For this review, take the finished solid that the model builds, in its own axes (mm). Coordinates: 2 decimals unless noted, no trailing zeros. Loops run counter-clockwise (first coordinate to the right, second up) from the corner with the lowest first, then second, coordinate; pieces in that order, holes last. Notation, with made-up numbers: M -29,61 L -5,61 A34 cw -5,100 Z; hole C 15,66.5 d8. An arc over 180 degrees is marked long. Put each result on its own line as item: value.
```python
from build123d import *

# Parameters (mm, degrees)
F1_DEPTH      = 3.414395
F1_DEPTH_BACK = 3.414395
F3_D          = 5.08
F3_DEPTH      = 38.1
F3_TIP        = 1.5261859723
F4_R          = 2.54


with BuildPart() as f1:
    # F0 (on Top) → F1 (new body, two sides)
    with BuildSketch(Plane.XY) as f1_sk:
        Polygon((27.5532683375, 33.9854207361), (8.2568451762, 33.9854207361), (8.2568451762, 27.1566307361), (62.6822561026, 27.1566307361), (81.9869935513, 27.1566307361), (81.9869935513, 33.9854207361), (78.0837014318, 33.9854207361), (71.3711140723, 33.9854207361), (58.8463247403, 33.9854207361), (56.5806804269, 33.9854207361), (53.2887220937, 33.9854207361), (51.0230777803, 33.9854207361), (45.4654522794, 33.9854207361), (43.199807966, 33.9854207361), (37.6421824652, 33.9854207361), (35.3765381518, 33.9854207361), (29.8189126509, 33.9854207361), align=None)
    extrude(amount=F1_DEPTH)
    extrude(f1_sk.sketch, amount=-F1_DEPTH_BACK)

    # F3
    with Locations(Plane.YZ.offset(81.9869935513)):
        with Locations((30.5710257361, 0)):
            Hole(F3_D / 2, depth=F3_DEPTH)
            with Locations((0, 0, -(F3_DEPTH + F3_TIP / 2))):  # 118° drill point
                Cone(0, F3_D / 2, F3_TIP, mode=Mode.SUBTRACT)

    # F4
    f4_edges = [f1.edges().sort_by_distance(p)[0] for p in [
        (45.121919, 33.985421, 3.414395),
        (45.121919, 27.156631, 3.414395),
        (45.121919, 33.985421, -3.414395),
        (45.121919, 27.156631, -3.414395),
    ]]
    fillet(f4_edges, radius=F4_R)


solid = f1.part
```
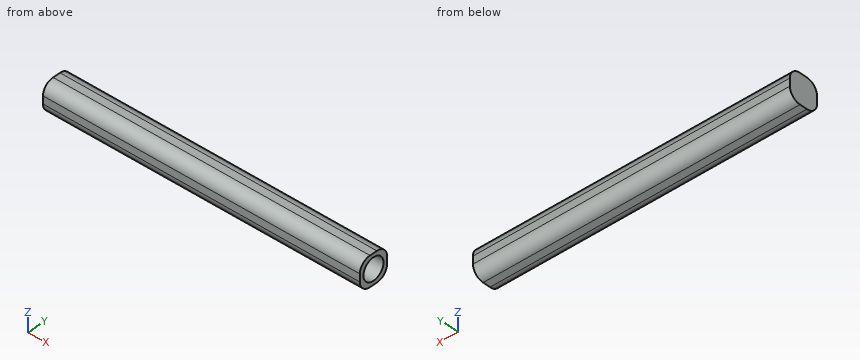
(1) Add section B-B (x = 39). Write out the cut boundary in (y, z), plus the area to 3 significant figures.
Determined:
outline: M 27.16,-0.87 A2.54 ccw 29.7,-3.41 L 31.45,-3.41 A2.54 ccw 33.99,-0.87 L 33.99,0.87 A2.54 ccw 31.45,3.41 L 29.7,3.41 A2.54 ccw 27.16,0.87 Z
area: 41.1 mm^2
(2) Wall thickness on line 1 along Z through (x, y) = (52.5, 30.75); line 2 along Y through (x, z) = (52, 0); line 3 along Y through (x, z) = (53.5, 1.5): over which ranges is each line inside the solid? List them lowest first. Write a range as [from, to].
Determined:
line 1: z = [-3.41, -2.53], [2.53, 3.41]
line 2: y = [27.16, 28.03], [33.11, 33.99]
line 3: y = [27.23, 28.52], [32.62, 33.91]
(3) Add section A-A (x = 66.5). Write out the cut boundary in (y, z).
Determined:
outline: M 27.16,-0.87 A2.54 ccw 29.7,-3.41 L 31.45,-3.41 A2.54 ccw 33.99,-0.87 L 33.99,0.87 A2.54 ccw 31.45,3.41 L 29.7,3.41 A2.54 ccw 27.16,0.87 Z; hole C 30.57,0 d5.08
(4) For pin 1 (4 mm diameter, centred on y = 30.57, z = 0, fed in from +X), flat-tipped, find the tip position at first contact; note if it passes through.
Determined:
pin 1: stops at x = 43.56
